```python
from build123d import *

# Parameters (mm, degrees)
SKETCH1_R           = 6.3627
SKETCH1_R_2         = 1.778
BOSS_EXTRUDE1_DEPTH = 2.286
SKETCH2_R           = 1.778
CUT_EXTRUDE1_DEPTH  = 7.62


with BuildPart() as part:
    # Sketch1 → Boss-Extrude1 (new body)
    with BuildSketch(Plane(origin=(0, 2.286, 0), x_dir=(1, 0, 0), z_dir=(0, 1, 0))):
        with BuildLine():
            Line((16.764, -35.060382), (16.764, 0))
            ThreePointArc((16.764, 0), (0, 16.764), (-16.764, 0))
            Line((-16.764, 0), (-16.764, -35.060382))
            ThreePointArc((-16.764, -35.060382), (-16.578012806, -35.509394806), (-16.129, -35.695382))
            Line((-16.129, -35.695382), (16.129, -35.695382))
            ThreePointArc((16.129, -35.695382), (16.578012806, -35.509394806), (16.764, -35.060382))
        make_face()
        with Locations(Location((0, 0, 0), (0, 0, 90))):
            Circle(SKETCH1_R, mode=Mode.SUBTRACT)
        with Locations(Location((9.779, 0, 0), (0, 0, 90))):
            Circle(SKETCH1_R_2, mode=Mode.SUBTRACT)
        with Locations(Location((6.914797213, 6.914797213, 0), (0, 0, 90))):
            Circle(SKETCH1_R_2, mode=Mode.SUBTRACT)
        with Locations(Location((0, 9.779, 0), (0, 0, 90))):
            Circle(SKETCH1_R_2, mode=Mode.SUBTRACT)
        with Locations(Location((-6.914797213, 6.914797213, 0), (0, 0, 90))):
            Circle(SKETCH1_R_2, mode=Mode.SUBTRACT)
        with Locations(Location((-9.779, 0, 0), (0, 0, 90))):
            Circle(SKETCH1_R_2, mode=Mode.SUBTRACT)
        with Locations(Location((-6.914797213, -6.914797213, 0), (0, 0, 90))):
            Circle(SKETCH1_R_2, mode=Mode.SUBTRACT)
        with Locations(Location((0, -9.779, 0), (0, 0, 90))):
            Circle(SKETCH1_R_2, mode=Mode.SUBTRACT)
        with Locations(Location((6.914797213, -6.914797213, 0), (0, 0, 90))):
            Circle(SKETCH1_R_2, mode=Mode.SUBTRACT)
        with Locations(Location((13.470384182, -32.520382, 0), (0, 0, 90))):
            Circle(SKETCH1_R_2, mode=Mode.SUBTRACT)
        with Locations(Location((-13.470384182, -32.520382, 0), (0, 0, 90))):
            Circle(SKETCH1_R_2, mode=Mode.SUBTRACT)
    extrude(amount=-BOSS_EXTRUDE1_DEPTH)

    # Sketch2 → Cut-Extrude1 (cut)
    with BuildSketch(Plane(origin=(0, 2.286, 0), x_dir=(1, 0, 0), z_dir=(0, 1, 0))):
        with Locations(Location((13.470384182, -19.820382, 0), (0, 0, 270))):
            Circle(SKETCH2_R)
        with Locations(Location((-13.470384182, -19.820382, 0), (0, 0, 270))):
            Circle(SKETCH2_R)
    extrude(amount=-CUT_EXTRUDE1_DEPTH, mode=Mode.SUBTRACT)


solid = part.part
```
The listing builds one solid part. Answer for the finished solid, in the listing's coordinates (mm). Round coordinates to 2 decimals unless told otherwise and drop trailing zeros. Loops run counter-clockwise (first coordinate to the right, second up) from the corner with the lowest first, then second, coordinate; pieces in that order, holes last.
Q1. Section A-A, the plane x = 0 is taken. Determine the outline of the cut face in (y, z), then the cut area to 3 significant figures.
Q2. Find the intervals of material crossed by line 1 (X direction, y = 0.5, z = 0); line 2 (Z direction, x = -12, y = 0.5); line 3 (Z direction, x = 14.5, y = 1.95), in increasing order.
Q3. Section C-C, the plane y = 1.35 is taken. Count the separate pieces of the cut face and the enclosed holes in it, then the cut area to 3 significant figures.
Q4. Section B-B, the plane z = -3 is taken. Determine the outline of the cut face in (x, y).
Q5. For a pull along X with two mould halves and no side action, classify faces 1 (the face through (16.764, 1, 18)), 2 (the face through (-13.392, 1.159, 18.044)), 3 (the face through (0, 1, 35.695)), 4 (the face through (0.37, 1.16, -16.76)) as released by +X, released by -X, zero draft, split by the parting line, or undercut.
Q6. Section D-D, the plane z = 7.5 is taken. Determine the outline of the cut face in (x, y), then the cut area to 3 significant figures.
Completed:
1. outline: (0, -16.76) - (2.29, -16.76) - (2.29, -11.56) - (0, -11.56) - close; (0, -8) - (2.29, -8) - (2.29, -6.36) - (0, -6.36) - close; (0, 6.36) - (2.29, 6.36) - (2.29, 8) - (0, 8) - close; (0, 11.56) - (2.29, 11.56) - (2.29, 35.7) - (0, 35.7) - close
1. area: 74.6 mm2
2. line 1: x = -16.76 to -11.56, -8 to -6.36, 6.36 to 8, 11.56 to 16.76
2. line 2: z = -11.71 to 18.82, 20.82 to 31.52, 33.52 to 35.7
2. line 3: z = -8.41 to 18.37, 21.27 to 31.07, 33.97 to 35.7
3. separate pieces: 1
3. enclosed holes: 13
3. area: 1,390 mm2
4. outline: (-16.49, 0) - (-5.61, 0) - (-5.61, 2.29) - (-16.49, 2.29) - close; (5.61, 0) - (16.49, 0) - (16.49, 2.29) - (5.61, 2.29) - close
5. face 1: released by +X
5. face 2: undercut
5. face 3: zero draft
5. face 4: split by the parting line
6. outline: (-16.76, 0) - (-8.59, 0) - (-8.59, 2.29) - (-16.76, 2.29) - close; (-5.24, 0) - (5.24, 0) - (5.24, 2.29) - (-5.24, 2.29) - close; (8.59, 0) - (16.76, 0) - (16.76, 2.29) - (8.59, 2.29) - close
6. area: 61.3 mm2
